Verification items for the finished model (mm, model axes). A direction names the side the tool comes from. Give positions to 0.01 mm unless a question says otherwise; leave off trailing zeros. Loops run counter-clockwise (first coordinate to the right, second up) from the corner with the lowest first, then second, coordinate; pieces in that order, holes last. Notation, with made-up numbers: M -12,26 L 39,26 A22 cw 39,33 Z; hole C -33,-18.5 d7. An arc over 180 degrees is marked long. Use a Markdown table: item, result.
from build123d import *

# Parameters (mm, degrees)
SKETCH_1_R          = 10.75
SKETCH_1_R_2        = 9
EXTRUDE_1_DEPTH     = 185
SKETCH_5_R          = 5
CUT_EXTRUDE_2_DEPTH = 10
SKETCH_6_R          = 1.058948346
CUT_EXTRUDE_3_DEPTH = 15


with BuildPart() as part:
    # 草图1 → 拉伸1 (new body)
    with BuildSketch(Plane(origin=(0, 0, 0), x_dir=(1, 0, 0), z_dir=(0, 1, 0))):
        with Locations(Location((0, 0, 0), (0, 0, 270))):
            Circle(SKETCH_1_R)
        with Locations(Location((0, 0, 0), (0, 0, 270))):
            Circle(SKETCH_1_R_2, mode=Mode.SUBTRACT)
    extrude(amount=EXTRUDE_1_DEPTH)

    # 草图3 → 旋转1 (revolve)
    with BuildSketch(Plane(origin=(0, 0, 0), x_dir=(0, 0, -1), z_dir=(1, 0, 0)), mode=Mode.PRIVATE) as revolve_1_sk:
        Polygon((0, 185), (-13, 185), (-13, 204), (-6, 204), (-6, 206), (0, 206), align=None)
    revolve(revolve_1_sk.sketch.rotate(Axis((0, 185, 0), (0, 1, 0)), 180), axis=Axis((0, 185, 0), (0, 1, 0)))

    # 草图4 → 旋转2 (revolve)
    with BuildSketch(Plane(origin=(0, 0, 0), x_dir=(0, 0, -1), z_dir=(1, 0, 0)), mode=Mode.PRIVATE) as revolve_2_sk:
        Polygon((5, 0), (13, 0), (13, -25), (6, -25), (6, -27), (5, -27), align=None)
    revolve(revolve_2_sk.sketch.rotate(Axis((0, 0, 0), (0, -1, 0)), 180), axis=Axis((0, 0, 0), (0, -1, 0)))

    # 草图5 → 拉伸2 (cut)
    with BuildSketch(Plane(origin=(13, 0, 0), x_dir=(0, 0, -1), z_dir=(1, 0, 0))):
        with Locations((0, 193)):
            Circle(SKETCH_5_R)
        with Locations((0, -8)):
            Circle(SKETCH_5_R)
    extrude(amount=-CUT_EXTRUDE_2_DEPTH, mode=Mode.SUBTRACT)

    # 草图6 → 拉伸3 (cut)
    with BuildSketch(Plane.XZ.offset(25)):
        with Locations(Location((7, 7, 0), (0, 0, 270))):
            Circle(SKETCH_6_R)
        with Locations(Location((-7, 7, 0), (0, 0, 270))):
            Circle(SKETCH_6_R)
        with Locations(Location((-7, -7, 0), (0, 0, 270))):
            Circle(SKETCH_6_R)
        with Locations(Location((7, -7, 0), (0, 0, 270))):
            Circle(SKETCH_6_R)
    extrude(amount=-CUT_EXTRUDE_3_DEPTH, mode=Mode.SUBTRACT)


solid = part.part
(1) Draft check along Y on faces 5 (the flat face through (3, 204, -6)), 6 (the flat face through (3, 193, 0)), 7 (the cylindrical face through (-1.802, -26.014, 5.723)). Enter one of: +Y half, -Y half, draft (parallel to the pull), parting line (faces both ways), or undercut.
Results below:
| item | result |
|---|---|
| face 5 | +Y half |
| face 6 | undercut |
| face 7 | draft |
(2) Cross-section at A-A on y = 26. Record the cut outline in (x, z).
Results below:
| item | result |
|---|---|
| outline | C 0,0 d21.5; hole C 0,0 d18 |
(3) Set-up check for faces 1 (the flat face through (-10, 185, -5)), 2 (the cylindrical face through (-1.802, 205.014, -5.723)), 3 (the flat face through (3, -25, 6)), 4 (the cylindrical face through (8.07, -6.5, -4.77)): record each of +Z, -Z, +X, -X, +Y, -Y from which the full face is reachable in a straight line by a thin tool's end or side.
Results below:
| item | result |
|---|---|
| face 1 | none |
| face 2 | +Y |
| face 3 | -Y |
| face 4 | +X |
(4) Material ranges on line 1 (Y direction, x = 2.25, z = 5.25); line 2 (X direction, y = -1, z = 0.5); line 3 (Y direction, x = 4.5, z = -3.25), recorded low to high.
Results below:
| item | result |
|---|---|
| line 1 | -27 to 0, 185 to 206 |
| line 2 | -12.99 to -4.97, 4.97 to 12.99 |
| line 3 | -27 to -11.8, -4.2 to 0, 185 to 189.2, 196.8 to 206 |
(5) Gauge pin test, flat ends, axial feed: P1, Ø12, axis at x = -9.5, y = 79, coming from the +Z side; P2, Ø1, axis at x = 6.5, z = 4, coming from the +Y side; P3, Ø1.1, axis at y = -8.5, z = -4.5, coming from the +X side. Record the tip position at first contact, or that the pin passes through.
Results below:
| item | result |
|---|---|
| P1 | z = 10.16 |
| P2 | y = 204 |
| P3 | x = 12.03 |
